```python
from build123d import *

# Parameters (mm, degrees)
FILLET1_R = 0.5


with BuildPart() as part:
    # Sketch1 → Revolve1 (revolve)
    with BuildSketch(Plane.XY, mode=Mode.PRIVATE) as revolve1_sk:
        with BuildLine():
            Line((0, 23), (0, 30.15))
            Line((0, 30.15), (5.7, 30.15))
            Line((5.7, 30.15), (9.05, 31.1))
            Line((9.05, 31.1), (10.15, 29.85))
            Line((10.15, 29.85), (10.15, 28.45))
            Line((10.15, 28.45), (6.813609391, 27.990655138))
            ThreePointArc((6.813609391, 27.990655138), (5.952260951, 27.067207064), (6.681984504, 26.036585399))
            Line((6.681984504, 26.036585399), (9.15, 25.35))
            Line((9.15, 25.35), (9.15, 22.95))
            Line((9.15, 22.95), (7.65, 21.9))
            Line((7.65, 21.9), (5.4, 23))
            Line((5.4, 23), (0, 23))
        make_face()
    revolve(revolve1_sk.sketch.rotate(Axis((0, 0, 0), (1, 0, 0)), 90), axis=Axis((0, 0, 0), (1, 0, 0)))

    # Fillet1
    fillet1_edges = [part.edges().sort_by_distance(p)[0] for p in [
        (0, 0, -30.15),
        (0, 0, -23),
    ]]
    fillet(fillet1_edges, radius=FILLET1_R)


solid = part.part
```
Check sheet for the modelled part. Datum: model origin and axes. Units: mm. A direction names the side the tool comes from. Coordinates: 2 decimals unless noted, no trailing zeros. Write each loop counter-clockwise with the first axis right and the second up, starting at its lowest first coordinate (ties: lowest second). Pieces come first, ordered by that corner, then holes. Notation, with made-up numbers: M 75.5,62 L 100.5,62 A14 ccw 100.5,70 Z; hole C 53,0.25 d6. An arc over 180 degrees is marked long. Use one line per item in the form item = value.
Item 1: Gauge pin test, flat ends, axial feed: pin 1 Ø12 at (y, z) = (-4, -16.5) entering from +X; pin 2 Ø4 at (x, z) = (3.5, 16) entering from +Y; pin 3 Ø6 at (x, y) = (6.5, 8.5) entering from -Z. Record the tip position at first contact, or that the pin passes through.
Answer below:
pin_1 = 9.15
pin_2 = 26.7
pin_3 = -30.33
Item 2: Set-up check for faces 4 (the face through (3.136, -29.893, -3.925)), 5 (the face through (0, -16, 18)): record each of +Z, -Z, +X, -X, +Y, -Y from which the full face is reachable in a straight line by a thin tool's end or side.
Answer below:
face_4 = -X
face_5 = +Z, -Z, -X, +Y, -Y
Item 3: Sectioned sample at C-C, the plane x = 1.75. Record the cut outline in (y, z), and give its area (3 significant figures).
Answer below:
outline = C 0,0 d60.3; hole C 0,0 d46
area = 1,190 mm^2
Item 4: Material ranges on L1, parallel to Y at x = 9, z = 5; L2, parallel to Y at x = 3.3, z = 0; L3, parallel to Y at x = 7, z = 6, recorded low to high. Write a range as from..to.
Answer below:
L1 = -30.68..-27.85, -24.89..-22.29, 22.29..24.89, 27.85..30.68
L2 = -30.15..-23, 23..30.15
L3 = -29.92..-27.37, -25.24..-21.39, 21.39..25.24, 27.37..29.92
Item 5: Release check for a two-part mould opening along Y. For faces 1 (the face through (9.15, -23, -4)), 2 (the face through (10.15, 24.2, 15.3)), 3 (the face through (5.91, 26.8, 13.94)) record: pulls with the +Y half, pulls with the -Y half, needs draft (parallel to the pull), parting line crosses it, or undercut.
Answer below:
face_1 = undercut
face_2 = needs draft
face_3 = parting line crosses it
Item 6: Sectioned sample at A-A, the plane y = 0. Record the cut outline in (x, z).
Answer below:
outline = M 0,-29.65 A0.5 ccw 0.5,-30.15 L 5.7,-30.15 L 9.05,-31.1 L 10.15,-29.85 L 10.15,-28.45 L 6.81,-27.99 A1 cw 6.68,-26.04 L 9.15,-25.35 L 9.15,-22.95 L 7.65,-21.9 L 5.4,-23 L 0.5,-23 A0.5 ccw 0,-23.5 Z; M 0,23.5 A0.5 ccw 0.5,23 L 5.4,23 L 7.65,21.9 L 9.15,22.95 L 9.15,25.35 L 6.68,26.04 A1 cw 6.81,27.99 L 10.15,28.45 L 10.15,29.85 L 9.05,31.1 L 5.7,30.15 L 0.5,30.15 A0.5 ccw 0,29.65 Z
